Could you check a few things on this model? Use its own coordinates, in mm. A direction names the side the tool comes from. Coordinates: 2 decimals unless noted, no trailing zeros. Loops run counter-clockwise (first coordinate to the right, second up) from the corner with the lowest first, then second, coordinate; pieces in that order, holes last.
Autodesk Inventor part; units mm, degrees
ref_plane "YZ Plane" through (0, 0, 0) normal (1, 0, 0) x (0, 1, 0)
ref_plane "XZ Plane" through (0, 0, 0) normal (0, 1, 0) x (-1, 0, 0)
ref_plane "XY Plane" through (0, 0, 0) normal (0, 0, 1) x (1, 0, 0)
sketch "Sketch1" plane through (0, 0, 0) normal (0, 1, 0) x (-1, 0, 0)
  line L0 (0, 0) -> (20, 0)
  line L1 (20, 0) -> (20, -60)
  line L2 (20, -60) -> (0, -60)
  line L3 (0, -60) -> (0, 0)
  dimension "d0" = 20
  dimension "d1" = 60
extrude "Extrusion1" add sketch "Sketch1" along normal blind 3
sketch "Sketch2" plane through (0, 3, 0) normal (0, 1, 0) x (1, 0, 0)
  line L0 (-20, 0) -> (0, 0)
  line L1 (0, 0) -> (-2, 0)
  line L2 (-2, 0) -> (-2, 60)
  line L3 (-2, 60) -> (0, 60)
  line L4 (0, 60) -> (0, 0)
  dimension "d4" = 2
  dimension "d5" = 60
extrude "Extrusion2" add sketch "Sketch2" along normal blind 10
sketch "Sketch3" plane through (0, 0, 0) normal (0, -1, 0) x (1, 0, 0)
  line L0 (-20, 0) -> (0, 0)
  line L1 (0, -60) -> (-20, -60)
  line L2 (-20, 0) -> (-14, 0)
  line L3 (-14, 0) -> (-14, -60)
  line L4 (-14, -60) -> (-20, -60)
  line L5 (-20, -60) -> (-20, 0)
  dimension "d8" = 6
extrude "Extrusion3" add sketch "Sketch3" along normal blind 20
sketch "Sketch4" plane through (-14, 0, 0) normal (1, 0, 0) x (0, 0, -1)
  line L0 (0, -20) -> (0, 3)
  line L1 (0, -8.5) -> (10, -8.5)
  line L2 (60, 0) -> (60, -20)
  circle A0 centre (10, -8.5) radius 3
  line L3 (60, -20) -> (0, -20)
  line L4 (0, -20) -> (60, -20)
  circle A1 centre (50, -8.5) radius 3
  point P0 (0, 0)
  dimension "d11" = 10
  dimension "d12" = 6
  dimension "d15" = 40
extrude "Extrusion4" cut sketch "Sketch4" against normal through all
fillet "Fillet1" radius 5 2 edges at (-20, 3, -30) (-14, 0, -30)
fillet "Fillet2" radius 3 2 edges at (-14, -20, -30) (-20, -20, -30)
fillet "Fillet3" radius 3 2 edges at (-2, 3, -30) (0, 0, -30)
fillet "Fillet4" radius 1 2 edges at (0, 13, -30) (-2, 13, -30)
sketch "Sketch5" plane through (-14, -5, 0) normal (1, 0, 0) x (0, 0, -1)
  line L0 (0, 0) -> (60, 0)
  line L1 (0, 0) -> (30, 0)
  line L2 (30, 0) -> (30, -7.5)
  line L3 (60, -15) -> (0, -15)
  line L4 (42.5, -15) -> (17.5, -15)
  line L5 (17.5, -15) -> (17.5, 0)
  line L6 (17.5, 0) -> (42.5, 0)
  line L7 (42.5, 0) -> (42.5, -15)
  line L8 (42.5, -15) -> (17.5, 0) construction
  line L9 (17.5, -15) -> (42.5, 0) construction
  point P0 (0, 5)
  dimension "d26" = 7.5
  dimension "d27" = 25
  dimension "d28" = 15
extrude "Extrusion5" cut sketch "Sketch5" against normal through all
fillet "Fillet5" radius 4 2 edges at (-17, -5, -42.5) (-17, -5, -17.5)
properties part number "CableChain_Holder"
(1) I need wall thicknesses on probe 1 along Y at (x, z) = (-8.75, -49.5); probe 2 along Y at (x, z) = (-16, -52); probe 3 along Y at (x, z) = (-17.9, -10). Which ranges of each line are inside material? Lowest first, please.
Answers:
probe 1: y = 0 to 3
probe 2: y = -19.83 to -10.74, -6.26 to 2.9
probe 3: y = -19.86 to -11.5, -5.5 to 2.07
(2) Which directions (+Z, -Z, +X, -X, +Y, -Y) give clear straight access to the entire face, cutting with the end or side of a thin tool? Please do faces 3 (the face through (-2, 9, -30)), 4 (the face through (-19.14, -19.1, -51.13)), 5 (the face through (-14, -12, -51)), 6 (the face through (-20, -4, -30)), 7 (the face through (-17.042, -6.203, -18.641)).
Answers:
face 3: +Z, -Z, -X, +Y
face 4: +Z, -Z, -X, -Y
face 5: +Z, -Z, +X, -Y
face 6: +Z, -Z, -X, +Y, -Y
face 7: +X, -X, -Y
(3) Imagine slicing it at D-D, the plane y = -3. Write out the boundary of the cut face in (x, z).
Answers:
outline: (-20, -60) - (-13.58, -60) - (-13.58, 0) - (-20, 0) - close
(4) Imagine slicing it at B-B, the plane x = -18. Write out the boundary of the cut face in (y, z), and give its area (3 significant figures).
Answers:
outline: (-19.83, -60) - (2, -60) - (2, 0) - (-19.83, 0) - (-19.83, -17.5) - (-9, -17.5) arc R4 cw to (-5, -21.5) - (-5, -38.5) arc R4 cw to (-9, -42.5) - (-19.83, -42.5) - close; hole circle Ø6 at (-8.5, -50); hole circle Ø6 at (-8.5, -10)
area: 889 mm2
(5) We'd pull the mould along Z, two halves only. Please class faces 1 (the face through (-0.9, 0.86, -29.58)), 2 (the face through (-16.96, -5.97, -11.61)): +Z half, -Z half, draft (parallel to the pull), parting line (faces both ways), or undercut.
Answers:
face 1: draft
face 2: undercut
(6) For pin 1 (1 mm diameter, centred on x = -9, z = -16.5, fed in from -Y); pin 2 (4 mm diameter, centred on x = -13.5, z = -36.5, fed in from +Y); pin 3 (5 mm diameter, centred on y = 10, z = -43, fed in from -X); pin 4 (5.5 mm diameter, centred on y = -8.5, z = -10, fed in from +X), each with a flat end and sliding along its axis, tell me the tip position at first contact or that it passes through.
Answers:
pin 1: stops at y = -0.03
pin 2: stops at y = 3
pin 3: stops at x = -2
pin 4: passes through
